Work out the finished part from the listing and answer in its coordinate system (mm). A direction names the side the tool comes from. Coordinates: 2 decimals unless noted, no trailing zeros. Loops run counter-clockwise (first coordinate to the right, second up) from the corner with the lowest first, then second, coordinate; pieces in that order, holes last. Notation, with made-up numbers: M -27,38.5 L 25,38.5 A8 cw 25,45.5 Z; hole C 86,-18 d3. An arc over 180 degrees is marked long. Write each question's results on one line, items separated by ' | '.
```python
from build123d import *

# Parameters (mm, degrees)
CYLINDER012_R     = 1.48
CYLINDER012_DEPTH = 12
EXTRUDE008_DEPTH  = 5
EXTRUDE_DEPTH     = 5


with BuildPart() as motorcoupler_couplershaft:
    # Cylinder012 → Cylinder012 (new body)
    with BuildSketch(Plane(origin=(-6, 2.5, 0), x_dir=(0, 0, -1), z_dir=(1, 0, 0))):
        Circle(CYLINDER012_R)
    extrude(amount=CYLINDER012_DEPTH)


with BuildPart() as motorcoupler_motorshaft:
    # Sketch008 → Extrude008 (new body)
    with BuildSketch(Plane(origin=(0, 0, 0), x_dir=(0, 0, -1), z_dir=(0, -1, 0))):
        with BuildLine():
            ThreePointArc((2.087463, -1.55), (2.6, 0), (2.087463, 1.55))
            Line((-2.087463, 1.55), (2.087463, 1.55))
            ThreePointArc((-2.087463, 1.55), (-2.6, 0), (-2.087463, -1.55))
            Line((-2.087463, -1.55), (2.087463, -1.55))
        make_face()
    extrude(amount=-EXTRUDE008_DEPTH)


with BuildPart() as motorcoupler:
    # Sketch007 → Extrude (new body)
    with BuildSketch(Plane.XZ):
        with BuildLine():
            Line((4.728709, -1.624596), (5.320013, 0))
            Line((5.320013, 0), (7.32185, 5.5))
            Line((-7.32185, 5.5), (7.32185, 5.5))
            Line((-5.320013, 0), (-7.32185, 5.5))
            Line((-4.728709, -1.624596), (-5.320013, 0))
            ThreePointArc((-4.728709, -1.624596), (-3.702087, -3.360737), (-2.073041, -4.55))
            Line((-2.073041, -4.55), (2.073041, -4.55))
            ThreePointArc((2.073041, -4.55), (3.702087, -3.360737), (4.728709, -1.624596))
        make_face()
    extrude(amount=-EXTRUDE_DEPTH)

    # Cut017: cut motorCoupler_motorShaft
    add(motorcoupler_motorshaft.part, mode=Mode.SUBTRACT)

    # Cut018: cut motorCoupler_couplerShaft
    add(motorcoupler_couplershaft.part, mode=Mode.SUBTRACT)


solid = motorcoupler.part
```
1) Given pin 1 Ø1.3 at (y, z) = (3, -1) entering from -X; pin 2 Ø1 at (y, z) = (1.5, -0.5) entering from +X, each flat-ended and moving along its own axis, determine where each tip first touches the part or whether it passes through.
Check result:
pin 1: x = -4.98 | pin 2: x = 5.22
2) For a pull along X with two mould halves and no side action, classify faces 1 (the face through (4, 2, -3)), 2 (the face through (0, 2.5, -2.6)), 3 (the face through (0, 2, -4.55)) as released by +X, released by -X, zero draft, split by the parting line, or undercut.
Check result:
face 1: released by +X | face 2: undercut | face 3: zero draft
3) Find section B-B, the plane x = 0. Give the vertices of the cut face in (y, z), and give its area (4 significant figures).
Check result:
outline: M 0,-4.55 L 5,-4.55 L 5,-2.6 L 0,-2.6 Z; M 0,2.6 L 5,2.6 L 5,5.5 L 0,5.5 Z | area: 24.25 mm^2
4) Find section A-A, the plane y = 4.2. Give the vertices of the cut face in (x, z), and give its area (3 significant figures).
Check result:
outline: M -7.32,5.5 L -5.32,0 L -4.73,-1.62 A5 ccw -2.07,-4.55 L 2.07,-4.55 A5 ccw 4.73,-1.62 L 5.32,0 L 7.32,5.5 Z; hole M -1.55,-2.09 A2.6 ccw 1.55,-2.09 L 1.55,2.09 A2.6 ccw -1.55,2.09 Z | area: 92.8 mm^2
5) Which of the six approach directions +Z, -Z, +X, -X, +Y, -Y give full straight-line access (tool end or side, diameter ignored) to faces 4 (the face through (0, 0, 3)), 5 (the face through (1.55, 1, 1))?
Check result:
face 4: +Z, -Z, +X, -X, -Y | face 5: +Y, -Y
6) Straight lines are drawn through the part: probe 1 along Y at (x, z) = (4.7, 0); probe 2 along X at (y, z) = (3.8, 2.25); probe 3 along Z at (x, y) = (0.5, 2.3). For each, find the intervals that lie inside material, in ascending order. Write a range as [from, to].
Check result:
probe 1: [0, 1.02], [3.98, 5] | probe 2: [-6.14, -1.3], [1.3, 6.14] | probe 3: [-4.55, -2.55], [2.55, 5.5]
7) Find section C-C, the plane x = 4. Give the vertices of the cut face in (y, z).
Check result:
outline: M 0,-3 L 5,-3 L 5,5.5 L 0,5.5 Z; hole C 2.5,0 d2.96
8) Find section D-D, the plane z = 0.25. Give the vertices of the cut face in (x, y).
Check result:
outline: M -5.41,0 L -1.55,0 L -1.55,1.04 L -5.41,1.04 Z; M -5.41,3.96 L -1.55,3.96 L -1.55,5 L -5.41,5 Z; M 1.55,0 L 5.41,0 L 5.41,1.04 L 1.55,1.04 Z; M 1.55,3.96 L 5.41,3.96 L 5.41,5 L 1.55,5 Z
